Source: CAD feature listing. Evaluate the final solid. Frame: model axes, mm. A direction names the side the tool comes from. Coordinates: 2 decimals unless noted, no trailing zeros. Loops run counter-clockwise (first coordinate to the right, second up) from the corner with the lowest first, then second, coordinate; pieces in that order, holes last. Notation, with made-up numbers: (22.5, 83.25) -> (62.5, 83.25) arc R26 ccw to (62.5, 120.25) -> close; hole circle Ø1 at (71.25, 75.25). An arc over 180 degrees is marked (long way). Answer as a JSON object with one key per item and string values. Group by question number.
Autodesk Inventor part; units mm, degrees
ref_plane "Work Plane1" through (-26.0554, 5.5841, 57.3172) normal (0, -1, 0) x (1, 0, 0)
ref_plane "Work Plane2" through (-31.4254, 8.4841, 38.2454) normal (0, -1, 0) x (1, 0, 0)
ref_plane "YZ Plane" through (0, 0, 0) normal (1, 0, 0) x (0, 1, 0)
ref_plane "Work Plane1" through (-26.0554, 5.5841, 57.3172) normal (0, -1, 0) x (1, 0, 0)
sketch "Sketch1" plane through (-26.0554, 5.5841, 57.3172) normal (0, -1, 0) x (1, 0, 0)
  arc A0 (-6.2529, -16.6318) -> (-5.7152, -17.8896) centre (-4.5084, -16.63) ccw
  line L0 (-6.2529, -16.6318) -> (-8.9554, -15.4715)
  arc A1 (-8.9554, -15.4715) -> (-9.6085, -15.4715) centre (-9.2819, -16.2321) ccw
  line L1 (-9.6085, -15.4715) -> (-11.5974, -15.1528)
  arc A2 (-11.5974, -15.1528) -> (-12.113, -13.8772) centre (-12.9119, -14.9421) ccw
  line L2 (-12.113, -13.8772) -> (-12.113, -11.7599)
  line L3 (-12.113, -11.7599) -> (-10.8096, -8.0503)
  line L4 (-10.8096, -8.0503) -> (-0.9192, -8.5103)
  arc A3 (-0.3314, -8.8426) -> (-0.9192, -8.5103) centre (-0.954, -9.258) ccw
  line L5 (-0.3314, -8.8426) -> (2.5309, -17.8896)
  arc A4 (2.5309, -18.6308) -> (2.5309, -17.8896) centre (1.3597, -18.2602) ccw
  line L6 (2.5309, -18.6308) -> (1.3597, -25.9399)
  line L7 (1.3597, -25.9399) -> (-2.6315, -30.1057)
  arc A5 (-3.5771, -30.3612) -> (-2.6315, -30.1057) centre (-3.3161, -29.4497) ccw
  line L8 (-3.5771, -30.3612) -> (-8.4584, -28.2656)
  arc A6 (-9.8385, -26.6044) -> (-8.4584, -28.2656) centre (-7.5216, -26.0835) ccw
  line L9 (-9.8385, -26.6044) -> (-9.8385, -22.4387)
  arc A7 (-9.6085, -21.9531) -> (-9.8385, -22.4387) centre (-9.2109, -22.4387) ccw
  line L10 (-9.6085, -21.9531) -> (-5.7152, -17.8896)
  line L11 (7.08, -38.1436) -> (-17.82, -38.1436)
  line L12 (7.08, 0) -> (7.08, -38.1436)
  line L13 (-17.12, 0) -> (7.08, 0)
  line L14 (-17.82, -38.1436) -> (-17.12, 0)
  line L15 (-15.12, 0) -> (-15.12, -2.1)
  line L16 (4.83, 0) -> (4.83, -2.3)
  line L17 (-7.5, -2.1) -> (-7.5, 0)
  line L18 (-5.08, 0) -> (-5.08, -2.1)
  line L19 (8.08, -39.1436) -> (-18.8385, -39.1436)
  line L20 (-18.8385, -39.1436) -> (-18.1018, 1)
  line L21 (-18.1018, 1) -> (8.08, 1)
  line L22 (8.08, 1) -> (8.08, -39.1436)
  line L23 (-18.8385, -39.1436) -> (-18.8385, 1)
  line L24 (-18.8385, 1) -> (-18.1018, 1)
  point P0 (26.0554, -57.3172)
  dimension "d2" = 1
extrude "Extrusion1" add sketch "Sketch1" along normal blind 0.5 contours L0 A1 L1 A2 L2 L3 L4 A3 L5 A4 L6 L7 A5 L8 A6 L9 A7 L10 A0 | L11 L14 L13 L12 | L19 L20 L21 L22 | L23 L24 L20
sketch "Sketch2" plane through (-26.0554, 5.5841, 57.3172) normal (0, 1, 0) x (1, 0, 0)
  line L0 (5.08, 0) -> (5.08, 2.1)
  line L1 (5.08, 2.1) -> (5.08, 0)
  line L2 (-5.08, 0) -> (-5.08, 2.1)
  line L3 (-7.5, 2.1) -> (-7.5, 0)
  line L4 (-15.12, 0) -> (-15.12, 2.1)
  line L5 (4.83, 2.3) -> (2.79, 2.3)
  line L6 (8.08, 39.1436) -> (8.08, -1)
  line L7 (-18.8385, 39.1436) -> (8.08, 39.1436)
  line L8 (5.08, 2.1) -> (5.08, 2.3)
  line L9 (5.08, 2.3) -> (4.83, 2.3)
  line L10 (2.79, 2.3) -> (-5.08, 2.3)
  line L11 (-5.08, 2.3) -> (-5.08, 2.0628)
  line L12 (-7.5, 2.1) -> (-7.5, 2.3)
  line L13 (-7.5, 2.3) -> (-15.12, 2.3)
  line L14 (-15.12, 2.3) -> (-15.12, 2.0628)
  line L15 (-7.5, 0) -> (-15.12, 0)
  line L16 (-5.08, 0) -> (5.08, 0)
  line L17 (8.08, -1) -> (-17.1109, -1)
  line L18 (-7.25, 2.55) -> (-15.37, 2.55)
  line L19 (-15.37, 2.55) -> (-15.37, -1)
  line L20 (-15.37, -1) -> (-7.25, -1)
  line L21 (-7.25, -1) -> (-7.25, 2.55)
  line L22 (-5.33, -1) -> (5.33, -1)
  line L23 (5.33, -1) -> (5.33, 2.55)
  line L24 (5.33, 2.55) -> (-5.33, 2.55)
  line L25 (-5.33, 2.55) -> (-5.33, -1)
  line L26 (8.08, -1) -> (-18.8385, -1)
  line L27 (-18.8385, -1) -> (-18.8385, 39.1436)
  line L28 (7.28, -0.2) -> (7.28, 38.3436)
  line L29 (7.28, 38.3436) -> (-18.0385, 38.3436)
  line L30 (-18.0385, 38.3436) -> (-18.0385, -0.2)
  line L31 (-18.0385, -0.2) -> (7.28, -0.2)
  point P0 (26.0554, 57.3172)
  point P1 (-5.33, -0.2)
  point P2 (-7.25, -0.2)
  point P3 (-7.25, -1)
  point P4 (-17.6109, -0.5)
  point P5 (-15.37, -0.2)
  point P6 (5.33, -0.2)
  point P7 (5.33, -1)
  point P8 (-17.1109, -1)
extrude "Extrusion2" add sketch "Sketch2" along normal blind 5.2 contours L6 L17 L23 L31 L28 L29 L30 L19 L26 L27 L7 | L17 L21 L31 L25
sketch "Sketch3" plane through (-17.9754, 5.0841, 58.3172) normal (1, 0, 0) x (0, 0, -1)
  line L0 (6.5, 4) -> (13.3, 4)
  line L1 (6.5, 7.65) -> (13.8, 7.65)
  line L2 (13.8, 7.65) -> (13.8, 3.5)
  line L3 (13.8, 3.5) -> (6.5, 3.5)
  line L4 (6.5, 3.5) -> (6.5, 7.65)
  line L5 (1, 3.4) -> (39.1436, 3.4)
  line L6 (39.1436, 3.4) -> (39.1436, 4)
  line L7 (13.3, 4) -> (39.1436, 4)
  line L8 (13.3, 4) -> (13.3, 7.15)
  line L9 (7, 7.15) -> (13.3, 7.15)
  line L10 (7, 4) -> (7, 7.15)
  line L11 (1, 4) -> (7, 4)
  line L12 (1, 3.4) -> (1, 4)
  point P0 (58.3172, -5.0841)
  dimension "d14" = 0.5
  dimension "d41" = 0.5
  dimension "d42" = 0.5
  dimension "d43" = 0.5
extrude "Extrusion3" cut sketch "Sketch3" against normal blind 5.2 contours L4 L1 L2 L7 L8 L9 L10 L0 | L0 L7 L2 L3 L4 | L10 L9 L8 L0
sketch "Sketch4" plane through (-26.0554, 10.7841, 57.3172) normal (0, 1, 0) x (1, 0, 0)
  line L0 (8.08, 5.5) -> (7.28, 5.5)
  line L1 (7.28, 5.5) -> (7.28, -0.2)
  line L2 (7.28, -0.2) -> (5.33, -0.2)
  line L3 (5.33, -0.2) -> (5.33, -1)
  line L4 (5.33, -1) -> (8.08, -1)
  line L5 (8.08, -1) -> (8.08, 5.5)
  line L6 (7.28, 12.8) -> (8.08, 12.8)
  line L7 (8.08, 12.8) -> (8.08, 39.1436)
  line L8 (8.08, 39.1436) -> (-18.8385, 39.1436)
  line L9 (-18.8385, 39.1436) -> (-18.8385, -1)
  line L10 (-18.8385, -1) -> (-15.37, -1)
  line L11 (-15.37, -1) -> (-15.37, -0.2)
  line L12 (-15.37, -0.2) -> (-18.0385, -0.2)
  line L13 (-18.0385, -0.2) -> (-18.0385, 38.3436)
  line L14 (-18.0385, 38.3436) -> (7.28, 38.3436)
  line L15 (7.28, 38.3436) -> (7.28, 12.8)
  line L16 (-7.25, -0.2) -> (-7.25, -1)
  line L17 (-7.25, -1) -> (-5.33, -1)
  line L18 (-5.33, -1) -> (-5.33, -0.2)
  line L19 (-5.33, -0.2) -> (-7.25, -0.2)
  line L20 (-15.37, -0.2) -> (-15.37, -1)
  line L21 (-15.37, -0.7) -> (-18.5385, -0.7)
  line L22 (-18.5385, -0.7) -> (-18.5385, 38.8436)
  line L23 (-18.5385, 38.8436) -> (7.78, 38.8436)
  line L24 (7.78, 38.8436) -> (7.78, 12.8)
  line L25 (7.78, 5.5) -> (7.78, -0.7)
  line L26 (7.78, -0.7) -> (5.33, -0.7)
  line L27 (-7.25, -0.7) -> (-5.33, -0.7)
  point P0 (8.08, 25.9718)
  point P1 (-15.37, -0.7)
  dimension "d44" = 0.3
  dimension "d45" = 0.3
  dimension "d46" = 0.3
  dimension "d47" = 0.3
  dimension "d48" = 0.3
  dimension "d49" = 0.3
extrude "Extrusion4" add sketch "Sketch4" along normal blind 1 contours L5 L4 L3 L26 L25 L0 | L24 L23 L22 L21 L11 L10 L9 L8 L7 L6 | L27 L18 L17 L16
sketch "Sketch5" plane through (-26.0554, 11.7841, 57.3172) normal (0, 1, 0) x (1, 0, 0)
  line L0 (-15.37, -1) -> (-15.37, -0.2)
  line L1 (8.08, 12.8) -> (8.08, 39.1436)
  line L2 (8.08, 39.1436) -> (-18.8385, 39.1436)
  line L3 (-18.8385, 39.1436) -> (-18.8385, -1)
  line L4 (-18.8385, -1) -> (-15.37, -1)
  line L5 (7.58, 5.5) -> (7.38, 5.5)
  line L6 (7.38, 5.5) -> (7.38, -0.3)
  line L7 (7.38, -0.3) -> (5.33, -0.3)
  line L8 (5.33, -0.3) -> (5.33, -0.5)
  line L9 (5.33, -0.5) -> (7.58, -0.5)
  line L10 (7.58, -0.5) -> (7.58, 5.5)
  line L11 (-7.25, -0.2) -> (-7.25, -1)
  line L12 (-7.25, -1) -> (-5.33, -1)
  line L13 (-15.37, -1) -> (-15.37, -0.2)
  line L14 (-15.37, -0.2) -> (-18.0385, -0.2)
  line L15 (-18.0385, -0.2) -> (-18.0385, 38.3436)
  line L16 (-18.0385, 38.3436) -> (7.28, 38.3436)
  line L17 (7.28, 38.3436) -> (7.28, 12.8)
  line L18 (-5.33, -0.2) -> (-7.25, -0.2)
  line L19 (-7.25, -0.2) -> (-7.25, -1)
  line L20 (7.28, 5.5) -> (7.28, -0.2)
  line L21 (7.28, -0.2) -> (5.33, -0.2)
  line L22 (-7.25, -0.2) -> (-7.25, -1)
  line L23 (-15.37, -1) -> (-15.37, -0.2)
  line L24 (-15.37, -0.2) -> (-18.0385, -0.2)
  line L25 (-18.0385, -0.2) -> (-18.0385, 38.3436)
  line L26 (-18.0385, 38.3436) -> (7.28, 38.3436)
  line L27 (-15.37, -1) -> (-15.37, -0.2)
  line L28 (-15.37, -0.2) -> (-18.0385, -0.2)
  line L29 (-18.0385, -0.2) -> (-18.0385, 38.3436)
  line L30 (-18.0385, 38.3436) -> (7.28, 38.3436)
  line L31 (7.28, 38.3436) -> (7.28, 12.8)
  line L32 (-7.25, -0.2) -> (-7.25, -1)
  line L33 (7.28, -0.2) -> (5.33, -0.2)
  line L34 (7.28, 12.8) -> (8.08, 12.8)
  line L35 (8.08, 12.8) -> (8.08, 39.1436)
  line L36 (8.08, 39.1436) -> (-18.8385, 39.1436)
  line L37 (-18.8385, 39.1436) -> (-18.8385, -1)
  line L38 (-18.8385, -1) -> (-15.37, -1)
  line L39 (8.08, -1) -> (8.08, 5.5)
  line L40 (8.08, 5.5) -> (7.28, 5.5)
  line L41 (7.28, 38.3436) -> (7.28, 12.8)
  line L42 (7.28, 12.8) -> (8.08, 12.8)
  line L43 (8.08, 12.8) -> (8.08, 39.1436)
  line L44 (8.08, 39.1436) -> (-18.8385, 39.1436)
  line L45 (-18.8385, 39.1436) -> (-18.8385, -1)
  line L46 (-18.8385, -1) -> (-15.37, -1)
  line L47 (8.08, -1) -> (8.08, 5.5)
  line L48 (8.08, 5.5) -> (7.28, 5.5)
  line L49 (7.28, 5.5) -> (7.28, -0.2)
  line L50 (7.28, 12.8) -> (8.08, 12.8)
  line L51 (8.08, 12.8) -> (8.08, 39.1436)
  line L52 (8.08, 39.1436) -> (-18.8385, 39.1436)
  line L53 (-18.8385, 39.1436) -> (-18.8385, -1)
  line L54 (-18.8385, -1) -> (-15.37, -1)
  line L55 (8.08, -1) -> (8.08, 5.5)
  line L56 (8.08, 5.5) -> (7.28, 5.5)
  line L57 (7.28, 5.5) -> (7.28, -0.2)
  line L58 (8.08, -1) -> (8.08, 5.5)
  line L59 (8.08, 5.5) -> (7.28, 5.5)
  line L60 (7.28, 5.5) -> (7.28, -0.2)
  line L61 (-5.33, -0.2) -> (-7.25, -0.2)
  line L62 (-7.25, -1) -> (-5.33, -1)
  line L63 (-5.33, -1) -> (-5.33, -0.2)
  line L64 (-5.33, -0.2) -> (-7.25, -0.2)
  line L65 (5.33, -0.2) -> (5.33, -1)
  line L66 (5.33, -1) -> (8.08, -1)
  line L67 (-7.25, -1) -> (-5.33, -1)
  line L68 (-5.33, -1) -> (-5.33, -0.2)
  line L69 (7.28, -0.2) -> (5.33, -0.2)
  line L70 (5.33, -0.2) -> (5.33, -1)
  line L71 (5.33, -1) -> (8.08, -1)
  line L72 (-7.25, -1) -> (-5.33, -1)
  line L73 (-5.33, -1) -> (-5.33, -0.2)
  line L74 (-5.33, -0.2) -> (-7.25, -0.2)
  line L75 (5.33, -0.2) -> (5.33, -1)
  line L76 (5.33, -1) -> (8.08, -1)
  line L77 (-5.33, -1) -> (-5.33, -0.2)
  line L78 (7.28, -0.2) -> (5.33, -0.2)
  line L79 (5.33, -0.2) -> (5.33, -1)
  line L80 (5.33, -1) -> (8.08, -1)
  line L81 (-15.37, -0.2) -> (-18.0385, -0.2)
  line L82 (-18.0385, -0.2) -> (-18.0385, 38.3436)
  line L83 (-18.0385, 38.3436) -> (7.28, 38.3436)
  line L84 (7.28, 38.3436) -> (7.28, 12.8)
  line L85 (7.28, 12.8) -> (8.08, 12.8)
  point P0 (26.0554, 57.3172)
extrude "Extrusion5" add sketch "Sketch5" along normal blind 0.6
chamfer "Chamfer1" distance 0.3 angle 45 7 edges at (-42.7597, 12.3841, 57.5172) (-44.0939, 12.3841, 38.2454) (-31.4347, 12.3841, 18.9736) (-18.7754, 12.3841, 31.7454) (-32.3454, 12.3841, 57.5172) (-18.7754, 12.3841, 54.6672) (-19.7504, 12.3841, 57.5172)
ref_plane "Work Plane2" through (-31.4254, 8.4841, 38.2454) normal (0, -1, 0) x (1, 0, 0)
sketch "Sketch6" plane through (-31.4254, 8.4841, 38.2454) normal (0, -1, 0) x (1, 0, 0)
  line L0 (-10, 19.2718) -> (-10, 20.0718)
  line L1 (-1.88, 20.0718) -> (-10, 20.0718)
  line L2 (-1.88, 20.0718) -> (-1.88, 19.2718)
  line L3 (-1.88, 19.2718) -> (0.04, 19.2718)
  line L4 (0.04, 19.2718) -> (0.04, 20.0718)
  line L5 (10.7, 20.0718) -> (0.04, 20.0718)
  line L6 (10.7, 20.0718) -> (10.7, 19.2718)
  line L7 (10.7, 19.2718) -> (12.65, 19.2718)
  line L8 (12.65, 19.2718) -> (12.65, -19.2718)
  line L9 (12.65, -19.2718) -> (-12.6685, -19.2718)
  line L10 (-12.6685, -19.2718) -> (-12.6685, 19.2718)
  line L11 (-12.6685, 19.2718) -> (-10, 19.2718)
  line L12 (-11.1685, -17.7718) -> (11.15, -17.7718)
  line L13 (11.15, -17.7718) -> (11.15, 17.7718)
  line L14 (11.15, 17.7718) -> (9.2, 17.7718)
  line L15 (9.2, 17.7718) -> (9.2, 18.5718)
  line L16 (9.2, 18.5718) -> (1.54, 18.5718)
  line L17 (1.54, 18.5718) -> (1.54, 17.7718)
  line L18 (1.54, 17.7718) -> (-3.38, 17.7718)
  line L19 (-3.38, 17.7718) -> (-3.38, 18.5718)
  line L20 (-3.38, 18.5718) -> (-8.5, 18.5718)
  line L21 (-8.5, 18.5718) -> (-8.5, 17.7718)
  line L22 (-8.5, 17.7718) -> (-11.1685, 17.7718)
  line L23 (-11.1685, 17.7718) -> (-11.1685, -17.7718)
  line L24 (-11.1685, 17.7718) -> (-11.1685, 19.2718)
  line L25 (11.15, 17.7718) -> (11.15, 19.2718)
  line L26 (-1.88, 19.2718) -> (-1.88, 17.7718)
  line L27 (0.04, 19.2718) -> (0.04, 17.7718)
  line L28 (11.15, -2.0718) -> (12.65, -2.0718)
  line L29 (12.65, -19.2718) -> (12.65, 6.2718)
  line L30 (11.15, 5.0718) -> (12.65, 5.0718)
  point P0 (31.4254, -38.2454)
  point P1 (12.45, 19.0718)
  point P2 (12.45, -19.0718)
  point P3 (12.65, 5.0718)
  point P4 (12.65, -2.0718)
  dimension "d50" = 1.5
  dimension "d51" = 17
  dimension "d52" = 14
extrude "Extrusion6" add sketch "Sketch6" along normal up to surface (2.9 mm away) contours L24 L23 L12 L13 L28 L8 L9 L10 L11 | L3 L27 L18 L26 | L30 L13 L25 L7 L8
fillet "Fillet2" radius 1 7 edges at (-42.5939, 5.5841, 38.9954) (-42.0097, 5.5841, 57.5172) (-32.3454, 5.5841, 56.0172) (-20.2754, 5.5841, 50.4172) (-18.7754, 5.5841, 39.7454) (-20.2754, 5.5841, 28.3236) (-31.4347, 5.5841, 20.4736)
equation "\"d45\" = d44"
equation "\"d46\" = d44"
equation "\"d47\" = d44"
equation "\"d49\" = d44"
properties part number "case"
1. Section query B-B on y = 7.5. Return loops of the section in (x, z), then the cut area to 3 significant figures.
2. Section query A-A on y = 10. Return loops of the section in (x, z), then the cut area to 3 significant figures.
3. Pin query (flat end, axial travel): pin 1 Ø5 at (x, z) = (-30.5, 43) entering from +Y; pin 2 Ø2 at (x, y) = (-29.5, 7.5) entering from +Z; pin 3 Ø0.7 at (x, z) = (-20, 55) entering from +Y. Return the tip coordinate at first contact, or that it passes through.
4. Section query C-C on x = -40.5. Return loops of the section in (y, z), then the cut area to 3 significant figures.
5. Section query D-D on z = 37. Return loops of the section in (x, y), then the cut area to 3 significant figures.
6. Ray query, L1, parallel to X at y = 12, z = 43; L2, parallel to Z at x = -20.5, y = 9; L3, parallel to Z at x = -19.25, y = 6.25. Return the intervals inside material, ascending.
7. Reachability of faces 1 (the face through (-19, 11, 58.017)), 2 (the face through (-43, 8.484, 31)), 3 (the face through (-33.305, 8, 57)) from +Z, -Z, +X, -X, +Y, -Y: full face, straight path, thin tool, end or side. Return the list, or none.
8. Mould query, pull axis X, two halves, no side actions, for faces 4 (the face through (-20.275, 8, 50)), 5 (the face through (-18.4, 10.1, 44.517)), 6 (the face through (-44.894, 9, 38)), 7 (the face through (-44.094, 10, 38)). Classes: pulls with the +X half, pulls with the -X half, needs draft (parallel to the pull), parting line crosses it, or undercut.
Solved:
{
 "1": {"outline": "(-44.89, 18.17) -> (-17.98, 18.17) -> (-17.98, 58.32) -> (-20.73, 58.32) -> (-20.73, 57.52) -> (-20.28, 57.52) -> (-20.28, 43.32) -> (-18.78, 43.32) -> (-18.78, 36.17) -> (-20.28, 36.17) -> (-20.28, 20.47) -> (-42.59, 20.47) -> (-42.59, 57.52) -> (-41.43, 57.52) -> (-41.43, 58.32) -> (-44.89, 58.32) -> close; (-33.31, 56.02) -> (-31.39, 56.02) -> (-31.39, 58.32) -> (-33.31, 58.32) -> close", "area": "231 mm^2"},
 "2": {"outline": "(-44.89, 18.17) -> (-17.98, 18.17) -> (-17.98, 44.52) -> (-18.78, 44.52) -> (-18.78, 18.97) -> (-44.09, 18.97) -> (-44.09, 57.52) -> (-41.43, 57.52) -> (-41.43, 58.32) -> (-44.89, 58.32) -> close; (-33.31, 57.52) -> (-31.39, 57.52) -> (-31.39, 58.32) -> (-33.31, 58.32) -> close; (-20.73, 57.52) -> (-18.78, 57.52) -> (-18.78, 51.82) -> (-17.98, 51.82) -> (-17.98, 58.32) -> (-20.73, 58.32) -> close", "area": "83.9 mm^2"},
 "3": {"pin 1": "y = 5.58", "pin 2": "z = 20.48", "pin 3": "y = 8.48"},
 "4": {"outline": "(5.08, 18.17) -> (12.38, 18.17) -> (12.38, 18.67) -> (12.08, 18.97) -> (11.78, 18.97) -> (11.78, 18.47) -> (10.78, 18.47) -> (10.78, 18.97) -> (8.48, 18.97) -> (8.48, 20.47) -> (6.58, 20.47) arc R1 cw to (5.58, 21.47) -> (5.58, 58.32) -> (5.08, 58.32) -> close", "area": "29.5 mm^2"},
 "5": {"outline": "(-44.89, 5.08) -> (-17.98, 5.08) -> (-17.98, 12.38) -> (-18.48, 12.38) -> (-18.78, 12.08) -> (-18.78, 11.78) -> (-18.28, 11.78) -> (-18.28, 10.78) -> (-18.78, 10.78) -> (-18.78, 6.58) arc R1 cw to (-19.78, 5.58) -> (-41.59, 5.58) arc R1 cw to (-42.59, 6.58) -> (-42.59, 8.48) -> (-44.09, 8.48) -> (-44.09, 10.78) -> (-44.59, 10.78) -> (-44.59, 11.78) -> (-44.09, 11.78) -> (-44.09, 12.08) -> (-44.39, 12.38) -> (-44.89, 12.38) -> close", "area": "28.0 mm^2"},
 "6": {"L1": "-44.89 to -44.09, -18.78 to -17.98", "L2": "18.17 to 18.97, 57.52 to 58.32", "L3": "18.17 to 36.17, 43.32 to 58.32"},
 "7": {"face 1": "none", "face 2": "+Y", "face 3": "+Z, +Y"},
 "8": {"face 4": "undercut", "face 5": "needs draft", "face 6": "pulls with the -X half", "face 7": "undercut"}
}
